Geometry check sheet. Reference: the model listing, model coordinates, mm. Give positions to 0.01 mm unless a question says otherwise; leave off trailing zeros. Loops run counter-clockwise (first coordinate to the right, second up) from the corner with the lowest first, then second, coordinate; pieces in that order, holes last. Notation, with made-up numbers: (27.25, 56) -> (76.25, 56) arc R25 cw to (76.25, 71) -> close; hole circle Ø3 at (71.25, -26.5). An arc over 180 degrees is marked (long way). Write item = value, one per line. Start each with the question number.
Autodesk Fusion 360 part; units mm, degrees
sketch "Sketch1" plane through (0, 0, 0) normal (0, 1, 0) x (1, 0, 0)
  line L0 (36.5192, 19.3301) -> (17.7088, 30.1903)
  line L1 (12.7088, 21.5301) -> (31.5192, 10.6699)
  arc A0 (31.5192, 10.6699) -> (36.5192, 19.3301) centre (34.0192, 15) ccw
  arc A1 (10.8333, -16.8119) -> (10.8333, 16.8119) centre (0, 0) ccw
  arc A2 (31.5192, 10.6699) -> (36.5192, 19.3301) centre (34.0192, 15) ccw
  arc A3 (12.7088, 21.5301) -> (10.8333, 16.8119) centre (60, 0) ccw
  line L2 (31.5192, -10.6699) -> (12.7088, -21.5301)
  arc A4 (36.5192, -19.3301) -> (31.5192, -10.6699) centre (34.0192, -15) ccw
  line L3 (17.7088, -30.1903) -> (36.5192, -19.3301)
  arc A5 (49.9762, -50.9855) -> (20.8572, -34.1736) centre (30, -51.9615) ccw
  line L4 (55, -30) -> (55, -51.7204)
  arc A6 (65, -30) -> (55, -30) centre (60, -30) ccw
  line L5 (65, -51.7204) -> (65, -30)
  arc A7 (99.1428, -34.1736) -> (70.0238, -50.9855) centre (90, -51.9615) ccw
  line L6 (83.4807, -19.3301) -> (102.2911, -30.1903)
  arc A8 (88.4807, -10.6699) -> (83.4807, -19.3301) centre (85.9807, -15) ccw
  line L7 (107.2911, -21.5301) -> (88.4807, -10.6699)
  arc A9 (109.1666, 16.8119) -> (109.1666, -16.8119) centre (120, 0) ccw
  line L8 (88.4807, 10.6699) -> (107.2911, 21.5301)
  arc A10 (83.4807, 19.3301) -> (88.4807, 10.6699) centre (85.9807, 15) ccw
  line L9 (102.2911, 30.1903) -> (83.4807, 19.3301)
  arc A11 (70.0238, 50.9855) -> (99.1428, 34.1736) centre (90, 51.9615) ccw
  line L10 (65, 30) -> (65, 51.7204)
  arc A12 (55, 30) -> (65, 30) centre (60, 30) ccw
  line L11 (55, 51.7204) -> (55, 30)
  arc A13 (20.8572, 34.1736) -> (49.9762, 50.9855) centre (30, 51.9615) ccw
  arc A14 (55, 51.7204) -> (49.9762, 50.9855) centre (60, 0) ccw
  arc A15 (20.8572, 34.1736) -> (17.7054, 30.1856) centre (60, 0) ccw
  arc A16 (70.0238, 50.9855) -> (65, 51.7204) centre (60, 0) ccw
  arc A17 (102.2911, 30.1903) -> (99.1428, 34.1736) centre (60, 0) ccw
  arc A18 (109.1666, 16.8119) -> (107.2911, 21.5301) centre (60, 0) ccw
  arc A19 (107.2911, -21.5301) -> (109.1666, -16.8119) centre (60, 0) ccw
  arc A20 (99.1428, -34.1736) -> (102.2911, -30.1903) centre (60, 0) ccw
  arc A21 (65, -51.7204) -> (70.0238, -50.9855) centre (60, 0) ccw
  arc A22 (49.9762, -50.9855) -> (55, -51.7204) centre (60, 0) ccw
  arc A23 (10.8333, -16.8119) -> (12.7088, -21.5301) centre (60, 0) ccw
  arc A24 (17.7088, -30.1903) -> (20.8572, -34.1736) centre (60, 0) ccw
  line L12 (60, 0) -> (62.25, 0)
  line L13 (62.25, 2.3452) -> (62.25, -2.3452)
  arc A25 (62.25, 2.3452) -> (62.25, -2.3452) centre (60, 0) ccw
  dimension "d5" = 360
extrude "Extrude1" add sketch "Sketch1" along normal blind 4
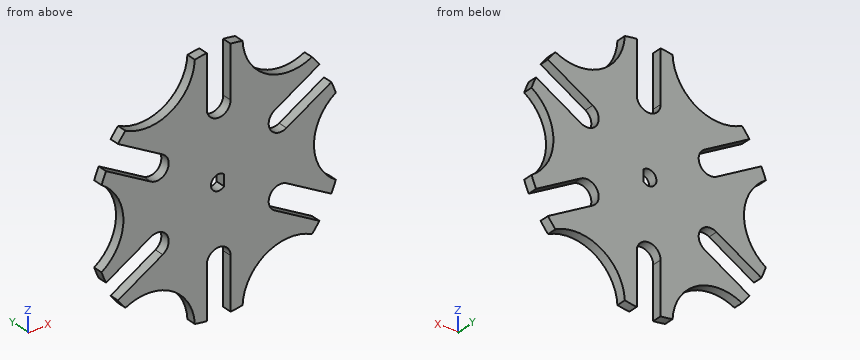
1) Section check C-C (x = 98). Enter the section's corners in (y, z).
2) Thickness scan on line 1 (X direction, y = 2.15, z = -34); line 2 (Z direction, x = 60, y = 1.9); line 3 (X direction, y = 0.35, z = 17). Record the ranges inside material, lowest first.
3) Depth check by flat-ended pin: pin 1 Ø2 at (x, y) = (99, 3) entering from +Z; pin 2 Ø2 at (y, z) = (1, 0.5) entering from -X; pin 3 Ø1.2 at (y, z) = (2.5, -39.5) entering from -X. Enter the tip coordinate at first touch or a pass-through.
4) Section check A-A (z = 0). Enter the section's corners in (x, y), plus the area to 3 significant figures.
5) Section check D-D (z = 15). Enter the section's corners in (x, y).
6) Section check B-B (x = 60). Enter the section's corners in (y, z), plus the area to 3 significant figures.
Check result:
q1.outline = (0, -33.63) -> (4, -33.63) -> (4, -27.71) -> (0, -27.71) -> close; (0, -16.17) -> (4, -16.17) -> (4, 16.17) -> (0, 16.17) -> close; (0, 27.71) -> (4, 27.71) -> (4, 33.63) -> (0, 33.63) -> close
q2.line_1 = 20.71 to 21.2, 38.8 to 55, 65 to 81.2, 98.8 to 99.29
q2.line_2 = -25 to -3.25, 3.25 to 25
q2.line_3 = 10.9 to 20.56, 38.6 to 81.4, 99.44 to 109.1
q3.pin_1 = 34.17
q3.pin_2 = 19.94
q3.pin_3 = 45.15
q4.outline = (20, 0) -> (56.75, 0) -> (56.75, 4) -> (20, 4) -> close; (62.25, 0) -> (100, 0) -> (100, 4) -> (62.25, 4) -> close
q4.area = 298 mm2
q5.outline = (13.23, 0) -> (24.02, 0) -> (24.02, 4) -> (13.23, 4) -> close; (39.02, 0) -> (80.98, 0) -> (80.98, 4) -> (39.02, 4) -> close; (95.98, 0) -> (106.77, 0) -> (106.77, 4) -> (95.98, 4) -> close
q6.outline = (0, -25) -> (4, -25) -> (4, -3.25) -> (0, -3.25) -> close; (0, 3.25) -> (4, 3.25) -> (4, 25) -> (0, 25) -> close
q6.area = 174 mm2
